Here's how the part is built. I have some questions about the finished solid (model axes, mm). A direction names the side the tool comes from. Round coordinates to 2 decimals unless told otherwise and drop trailing zeros. Loops run counter-clockwise (first coordinate to the right, second up) from the corner with the lowest first, then second, coordinate; pieces in that order, holes last. Notation, with made-up numbers: (-19.75, 58.5) - (23.25, 58.5) arc R13 ccw to (23.25, 69.5) - close; hole circle Ø6 at (34.5, 1). An arc over 180 degrees is marked (long way). Answer as a JSON object with one key per item and string values. Group by question number.
1) I want a section at D-D, the plane y = -2.25. Please give me the cut outline in (x, z).
2) Will these pins go through, and if not, where does the flat tip stop? P1, Ø1.6, axis at y = -9.5, z = 13, coming from the -X side; P2, Ø3, axis at y = -11.5, z = 12.5, coming from the +X side.
3) I want a section at A-A, the plane y = -10. Give the number of separate pieces and of enclosed holes in the cut face, then the cut area to 3 significant figures.
4) If we mould it in two halves opening along X, with no side actions, what happens to faces 1 (the face through (0, -10, -22)), 2 (the face through (23, -14, 5.5)), 3 (the face through (-17, -10, 13))? For each: pulls with the +X half, pulls with the -X half, needs draft (parallel to the pull), parting line crosses it, or undercut.
5) If I drill on line 1 along Z through (x, y) = (23, -5.5); line 2 along Z through (x, y) = (23, -3.25); line 3 along X through (y, z) = (-7.25, -3), over which ranges is the centre line in solid material (lowest first)? Write a range as [from, to].
6) I want a section at B-B, the plane x = 0. Please give me the cut outline in (y, z).
7) Which directions (+Z, -Z, +X, -X, +Y, -Y) give clear straight access to the entire face, cutting with the end or side of a thin tool? Please do faces 4 (the face through (28.4, -7.6, 10.5)), 5 (the face through (-17.6, -7.6, 10.5)), 6 (the face through (25.49, -14.79, 8.04)).
8) I want a section at C-C, the plane z = -15. Please give me the cut outline in (x, y).
from build123d import *

# Parameters (mm, degrees)
F0_R           = 2.75
F0_R_2         = 4
F1_DEPTH       = 20
F2_SIZE        = 1
F4_D           = 6.6
F4_CBORE_D     = 10.8
F4_CBORE_DEPTH = 5


with BuildPart() as f1:
    # F0 (on Front) → F1 (new body)
    with BuildSketch(Plane.XZ):
        Polygon((17, 17), (-17, 17), (-17, 10.5), (-30, 10.5), (-30, -22), (30, -22), (30, 10.5), (17, 10.5), align=None)
        with Locations((-23, -15)):
            Circle(F0_R, mode=Mode.SUBTRACT)
        with Locations((23, -15)):
            Circle(F0_R, mode=Mode.SUBTRACT)
        with Locations((-23, 0)):
            Circle(F0_R, mode=Mode.SUBTRACT)
        Circle(F0_R_2, mode=Mode.SUBTRACT)
        with Locations((23, 0)):
            Circle(F0_R, mode=Mode.SUBTRACT)
    extrude(amount=F1_DEPTH)

    # F2
    f2_edges = [f1.edges().sort_by_distance(p)[0] for p in [
        (17, -10, 17),
        (-17, -10, 17),
        (30, -10, 10.5),
        (-30, -10, 10.5),
    ]]
    chamfer(f2_edges, length=F2_SIZE)

    # F4 (through all)
    with Locations(Plane.XY.offset(10.5)):
        with Locations((-23, -10), (23, -10)):
            CounterBoreHole(F4_D / 2, F4_CBORE_D / 2, F4_CBORE_DEPTH)


solid = f1.part
Outcome:
{
 "1": {"outline": "(-30, -22) - (30, -22) - (30, 9.5) - (29, 10.5) - (17, 10.5) - (17, 16) - (16, 17) - (-16, 17) - (-17, 16) - (-17, 10.5) - (-29, 10.5) - (-30, 9.5) - close; hole circle Ø5.5 at (-23, -15); hole circle Ø5.5 at (-23, 0); hole circle Ø8 at (0, 0); hole circle Ø5.5 at (23, -15); hole circle Ø5.5 at (23, 0)"},
 "2": {"P1": "x = -17", "P2": "x = 17"},
 "3": {"separate pieces": "3", "enclosed holes": "1", "area": "1,650 mm^2"},
 "4": {"face 1": "needs draft", "face 2": "undercut", "face 3": "pulls with the -X half"},
 "5": {"line 1": "[-22, -17.75], [-12.25, -2.75], [2.75, 5.5]", "line 2": "[-22, -17.75], [-12.25, -2.75], [2.75, 10.5]", "line 3": "[-30, -24.82], [-21.18, -2.65], [2.65, 21.18], [24.82, 30]"},
 "6": {"outline": "(-20, -22) - (0, -22) - (0, -4) - (-20, -4) - close; (-20, 4) - (0, 4) - (0, 17) - (-20, 17) - close"},
 "7": {"face 4": "+Z, +X, +Y, -Y", "face 5": "+Z, -X, +Y, -Y", "face 6": "+Z"},
 "8": {"outline": "(-30, -20) - (-25.75, -20) - (-25.75, -11.82) arc R3.3 cw to (-25.75, -8.18) - (-25.75, 0) - (-30, 0) - close; (-20.25, -20) - (20.25, -20) - (20.25, -11.82) arc R3.3 cw to (20.25, -8.18) - (20.25, 0) - (-20.25, 0) - (-20.25, -8.18) arc R3.3 cw to (-20.25, -11.82) - close; (25.75, -20) - (30, -20) - (30, 0) - (25.75, 0) - (25.75, -8.18) arc R3.3 cw to (25.75, -11.82) - close"}
}
